Here's how the part is built. I have some questions about the finished solid (model axes, mm). Coordinates: 2 decimals unless noted, no trailing zeros. Write each loop counter-clockwise with the first axis right and the second up, starting at its lowest first coordinate (ties: lowest second). Pieces come first, ordered by that corner, then holes. Notation, with made-up numbers: (-11, 31) - (32, 31) arc R24 ccw to (32, 57) - close; hole circle Ø3 at (29, -40). An arc over 180 degrees is marked (long way). Answer in a Markdown table with one row per item. Add a question column.
Item 1: Imagine slicing it at C-C (y = 3.1). State how many separate pieces and enclosed holes the cut face has, plus the area to 3 significant figures.
Item 2: Imagine slicing it at A-A (x = 41.5). Please give me the cut outline in (y, z).
Item 3: If I drill on probe 1 along X at (y, z) = (2.25, 0); probe 2 along X at (y, z) = (2, 75); probe 3 along X at (y, z) = (3.3, -32), over which ranges is the centre line in solid material (lowest first)? Write a range as from..to.
Item 4: Imagine slicing it at B-B (z = -16.5). Please give me the cut outline in (x, y).
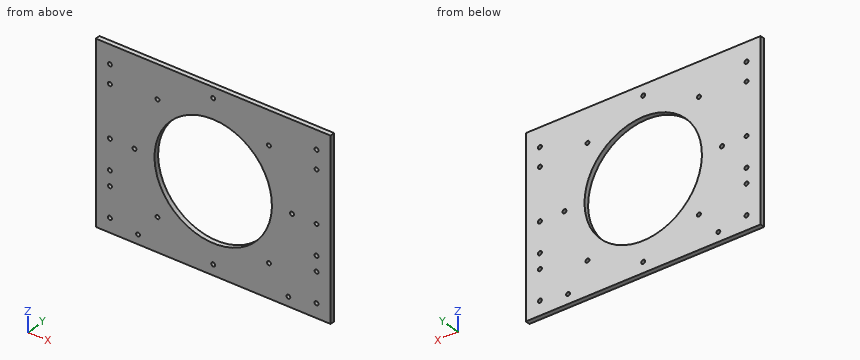
from build123d import *

# Parameters (mm, degrees)
SKETCH_1_W           = 250
SKETCH_1_H           = 190
EXTRUDE_1_DEPTH      = 5
SKETCH_2_R           = 2.1
CUT_EXTRUDE_1_DEPTH  = 10
SKETCH_3_R           = 62.5
CUT_EXTRUDE_2_DEPTH  = 10
CUT_EXTRUDE_3_REACH  = 159.083
SKETCH_4_R           = 2.1
SKETCH_5_OUTSIDE_W   = 314.81
SKETCH_5_OUTSIDE_H   = 254.81
SKETCH_5_OUTSIDE_W_2 = 250
SKETCH_5_OUTSIDE_H_2 = 190
SKETCH_5_OUTSIDE_R   = 2.05
CUT_EXTRUDE_4_DEPTH  = 10


with BuildPart() as part:
    # 草图1 → 凸台-拉伸1 (new body)
    with BuildSketch(Plane(origin=(0, 0, 0), x_dir=(1, 0, 0), z_dir=(0, 1, 0))):
        Rectangle(SKETCH_1_W, SKETCH_1_H)
    extrude(amount=EXTRUDE_1_DEPTH)

    # 草图2 → 切除-拉伸1 (cut)
    with BuildSketch(Plane(origin=(0, 5, 0), x_dir=(1, 0, 0), z_dir=(0, 1, 0))):
        with Locations(Location((-83.9, 0, 0), (0, 0, 270))):
            Circle(SKETCH_2_R)
        with Locations(Location((-59.326258942, 59.326258942, 0), (0, 0, 270))):
            Circle(SKETCH_2_R)
        with Locations(Location((0, 83.9, 0), (0, 0, 270))):
            Circle(SKETCH_2_R)
        with Locations(Location((59.326258942, 59.326258942, 0), (0, 0, 270))):
            Circle(SKETCH_2_R)
        with Locations(Location((83.9, 0, 0), (0, 0, 270))):
            Circle(SKETCH_2_R)
        with Locations(Location((59.326258942, -59.326258942, 0), (0, 0, 270))):
            Circle(SKETCH_2_R)
        with Locations(Location((0, -83.9, 0), (0, 0, 270))):
            Circle(SKETCH_2_R)
        with Locations(Location((-59.326258942, -59.326258942, 0), (0, 0, 270))):
            Circle(SKETCH_2_R)
    extrude(amount=-CUT_EXTRUDE_1_DEPTH, mode=Mode.SUBTRACT)

    # 草图3 → 切除-拉伸2 (cut)
    with BuildSketch(Plane(origin=(0, 5, 0), x_dir=(1, 0, 0), z_dir=(0, 1, 0))):
        with Locations(Location((0, 0, 0), (0, 0, 270))):
            Circle(SKETCH_3_R)
    extrude(amount=-CUT_EXTRUDE_2_DEPTH, mode=Mode.SUBTRACT)

    # 草图4 → 切除-拉伸3 (cut, up to next)
    with BuildSketch(Plane(origin=(0, 5, 0), x_dir=(1, 0, 0), z_dir=(0, 1, 0)), mode=Mode.PRIVATE) as cut_extrude_3_sk1:
        with Locations(Location((-110, 80, 0), (0, 0, 270))):
            Circle(SKETCH_4_R)
    cut_extrude_3_tool1 = extrude(cut_extrude_3_sk1.sketch, amount=-CUT_EXTRUDE_3_REACH, mode=Mode.PRIVATE) & part.part
    # 草图4 → 切除-拉伸3 (cut, up to next)
    with BuildSketch(Plane(origin=(0, 5, 0), x_dir=(1, 0, 0), z_dir=(0, 1, 0)), mode=Mode.PRIVATE) as cut_extrude_3_sk2:
        with Locations(Location((-110, 48, 0), (0, 0, 270))):
            Circle(SKETCH_4_R)
    cut_extrude_3_tool2 = extrude(cut_extrude_3_sk2.sketch, amount=-CUT_EXTRUDE_3_REACH, mode=Mode.PRIVATE) & part.part
    # 草图4 → 切除-拉伸3 (cut, up to next)
    with BuildSketch(Plane(origin=(0, 5, 0), x_dir=(1, 0, 0), z_dir=(0, 1, 0)), mode=Mode.PRIVATE) as cut_extrude_3_sk3:
        with Locations(Location((110, 48, 0), (0, 0, 270))):
            Circle(SKETCH_4_R)
    cut_extrude_3_tool3 = extrude(cut_extrude_3_sk3.sketch, amount=-CUT_EXTRUDE_3_REACH, mode=Mode.PRIVATE) & part.part
    # 草图4 → 切除-拉伸3 (cut, up to next)
    with BuildSketch(Plane(origin=(0, 5, 0), x_dir=(1, 0, 0), z_dir=(0, 1, 0)), mode=Mode.PRIVATE) as cut_extrude_3_sk4:
        with Locations(Location((110, 80, 0), (0, 0, 270))):
            Circle(SKETCH_4_R)
    cut_extrude_3_tool4 = extrude(cut_extrude_3_sk4.sketch, amount=-CUT_EXTRUDE_3_REACH, mode=Mode.PRIVATE) & part.part
    # 草图4 → 切除-拉伸3 (cut, up to next)
    with BuildSketch(Plane(origin=(0, 5, 0), x_dir=(1, 0, 0), z_dir=(0, 1, 0)), mode=Mode.PRIVATE) as cut_extrude_3_sk5:
        with Locations(Location((-110, -75, 0), (0, 0, 270))):
            Circle(SKETCH_4_R)
    cut_extrude_3_tool5 = extrude(cut_extrude_3_sk5.sketch, amount=-CUT_EXTRUDE_3_REACH, mode=Mode.PRIVATE) & part.part
    # 草图4 → 切除-拉伸3 (cut, up to next)
    with BuildSketch(Plane(origin=(0, 5, 0), x_dir=(1, 0, 0), z_dir=(0, 1, 0)), mode=Mode.PRIVATE) as cut_extrude_3_sk6:
        with Locations(Location((110, -75, 0), (0, 0, 270))):
            Circle(SKETCH_4_R)
    cut_extrude_3_tool6 = extrude(cut_extrude_3_sk6.sketch, amount=-CUT_EXTRUDE_3_REACH, mode=Mode.PRIVATE) & part.part
    # 草图4 → 切除-拉伸3 (cut, up to next)
    with BuildSketch(Plane(origin=(0, 5, 0), x_dir=(1, 0, 0), z_dir=(0, 1, 0)), mode=Mode.PRIVATE) as cut_extrude_3_sk7:
        with Locations(Location((-110, 32, 0), (0, 0, 270))):
            Circle(SKETCH_4_R)
    cut_extrude_3_tool7 = extrude(cut_extrude_3_sk7.sketch, amount=-CUT_EXTRUDE_3_REACH, mode=Mode.PRIVATE) & part.part
    # 草图4 → 切除-拉伸3 (cut, up to next)
    with BuildSketch(Plane(origin=(0, 5, 0), x_dir=(1, 0, 0), z_dir=(0, 1, 0)), mode=Mode.PRIVATE) as cut_extrude_3_sk8:
        with Locations(Location((-110, 0, 0), (0, 0, 270))):
            Circle(SKETCH_4_R)
    cut_extrude_3_tool8 = extrude(cut_extrude_3_sk8.sketch, amount=-CUT_EXTRUDE_3_REACH, mode=Mode.PRIVATE) & part.part
    # 草图4 → 切除-拉伸3 (cut, up to next)
    with BuildSketch(Plane(origin=(0, 5, 0), x_dir=(1, 0, 0), z_dir=(0, 1, 0)), mode=Mode.PRIVATE) as cut_extrude_3_sk9:
        with Locations(Location((110, 32, 0), (0, 0, 270))):
            Circle(SKETCH_4_R)
    cut_extrude_3_tool9 = extrude(cut_extrude_3_sk9.sketch, amount=-CUT_EXTRUDE_3_REACH, mode=Mode.PRIVATE) & part.part
    # 草图4 → 切除-拉伸3 (cut, up to next)
    with BuildSketch(Plane(origin=(0, 5, 0), x_dir=(1, 0, 0), z_dir=(0, 1, 0)), mode=Mode.PRIVATE) as cut_extrude_3_sk10:
        with Locations(Location((110, 0, 0), (0, 0, 270))):
            Circle(SKETCH_4_R)
    cut_extrude_3_tool10 = extrude(cut_extrude_3_sk10.sketch, amount=-CUT_EXTRUDE_3_REACH, mode=Mode.PRIVATE) & part.part
    # 草图4 → 切除-拉伸3 (cut, up to next)
    with BuildSketch(Plane(origin=(0, 5, 0), x_dir=(1, 0, 0), z_dir=(0, 1, 0)), mode=Mode.PRIVATE) as cut_extrude_3_sk11:
        with Locations(Location((-110, -55, 0), (0, 0, 270))):
            Circle(SKETCH_4_R)
    cut_extrude_3_tool11 = extrude(cut_extrude_3_sk11.sketch, amount=-CUT_EXTRUDE_3_REACH, mode=Mode.PRIVATE) & part.part
    # 草图4 → 切除-拉伸3 (cut, up to next)
    with BuildSketch(Plane(origin=(0, 5, 0), x_dir=(1, 0, 0), z_dir=(0, 1, 0)), mode=Mode.PRIVATE) as cut_extrude_3_sk12:
        with Locations(Location((110, -55, 0), (0, 0, 270))):
            Circle(SKETCH_4_R)
    cut_extrude_3_tool12 = extrude(cut_extrude_3_sk12.sketch, amount=-CUT_EXTRUDE_3_REACH, mode=Mode.PRIVATE) & part.part
    add(cut_extrude_3_tool1.solids().sort_by_distance((-110, 5, -80))[0], mode=Mode.SUBTRACT)
    add(cut_extrude_3_tool2.solids().sort_by_distance((-110, 5, -48))[0], mode=Mode.SUBTRACT)
    add(cut_extrude_3_tool3.solids().sort_by_distance((110, 5, -48))[0], mode=Mode.SUBTRACT)
    add(cut_extrude_3_tool4.solids().sort_by_distance((110, 5, -80))[0], mode=Mode.SUBTRACT)
    add(cut_extrude_3_tool5.solids().sort_by_distance((-110, 5, 75))[0], mode=Mode.SUBTRACT)
    add(cut_extrude_3_tool6.solids().sort_by_distance((110, 5, 75))[0], mode=Mode.SUBTRACT)
    add(cut_extrude_3_tool7.solids().sort_by_distance((-110, 5, -32))[0], mode=Mode.SUBTRACT)
    add(cut_extrude_3_tool8.solids().sort_by_distance((-110, 5, 0))[0], mode=Mode.SUBTRACT)
    add(cut_extrude_3_tool9.solids().sort_by_distance((110, 5, -32))[0], mode=Mode.SUBTRACT)
    add(cut_extrude_3_tool10.solids().sort_by_distance((110, 5, 0))[0], mode=Mode.SUBTRACT)
    add(cut_extrude_3_tool11.solids().sort_by_distance((-110, 5, 55))[0], mode=Mode.SUBTRACT)
    add(cut_extrude_3_tool12.solids().sort_by_distance((110, 5, 55))[0], mode=Mode.SUBTRACT)

    # 草图5 outside → 切除-拉伸4 (cut)
    # profile 1 of 3: a face of its own
    with BuildSketch(Plane(origin=(0, 5, 0), x_dir=(1, 0, 0), z_dir=(0, 1, 0))):
        Rectangle(SKETCH_5_OUTSIDE_W, SKETCH_5_OUTSIDE_H)
        Rectangle(SKETCH_5_OUTSIDE_W_2, SKETCH_5_OUTSIDE_H_2, mode=Mode.SUBTRACT)
    # profile 2 of 3: a face of its own
    with BuildSketch(Plane(origin=(0, 5, 0), x_dir=(1, 0, 0), z_dir=(0, 1, 0))):
        with Locations(Location((-80, 85, 0), (0, 0, 270))):
            Circle(SKETCH_5_OUTSIDE_R)
    # profile 3 of 3: a face of its own
    with BuildSketch(Plane(origin=(0, 5, 0), x_dir=(1, 0, 0), z_dir=(0, 1, 0))):
        with Locations(Location((80, 85, 0), (0, 0, 270))):
            Circle(SKETCH_5_OUTSIDE_R)
    extrude(amount=-CUT_EXTRUDE_4_DEPTH, mode=Mode.SUBTRACT)


solid = part.part
Here are the results:
| question | item | result |
|---|---|---|
| 1 | separate pieces | 1 |
| 1 | enclosed holes | 23 |
| 1 | area | 34,900 mm2 |
| 2 | outline | (0, -95) - (5, -95) - (5, -46.73) - (0, -46.73) - close; (0, 46.73) - (5, 46.73) - (5, 95) - (0, 95) - close |
| 3 | probe 1 | x = -125..-112.1, -107.9..-86, -81.8..-62.5, 62.5..81.8, 86..107.9, 112.1..125 |
| 3 | probe 2 | x = -125..-112.1, -107.9..107.9, 112.1..125 |
| 3 | probe 3 | x = -125..-112.1, -107.9..-53.69, 53.69..107.9, 112.1..125 |
| 4 | outline | (-125, 0) - (-60.28, 0) - (-60.28, 5) - (-125, 5) - close; (60.28, 0) - (125, 0) - (125, 5) - (60.28, 5) - close |
